Geometry check sheet. Reference: drawing and pictorial views, mm from the part's lowest x, y, z. A direction names the side the tool comes from. Give positions to 0.01 mm unless a question says otherwise; leave off trailing zeros. Order: outer loops, then holes, each group sorted by start corner. A loop starts at its lowest first (then second) coordinate and runs counter-clockwise, first axis right, second up. Notation, with made-up numbers: (68.5, 74.5) - (88.5, 74.5) arc R23 cw to (88.5, 82.5) - close; hole circle Ø3 at (7, 47). An arc over 180 degrees is marked (long way). Answer in a Markdown table with one row per item.
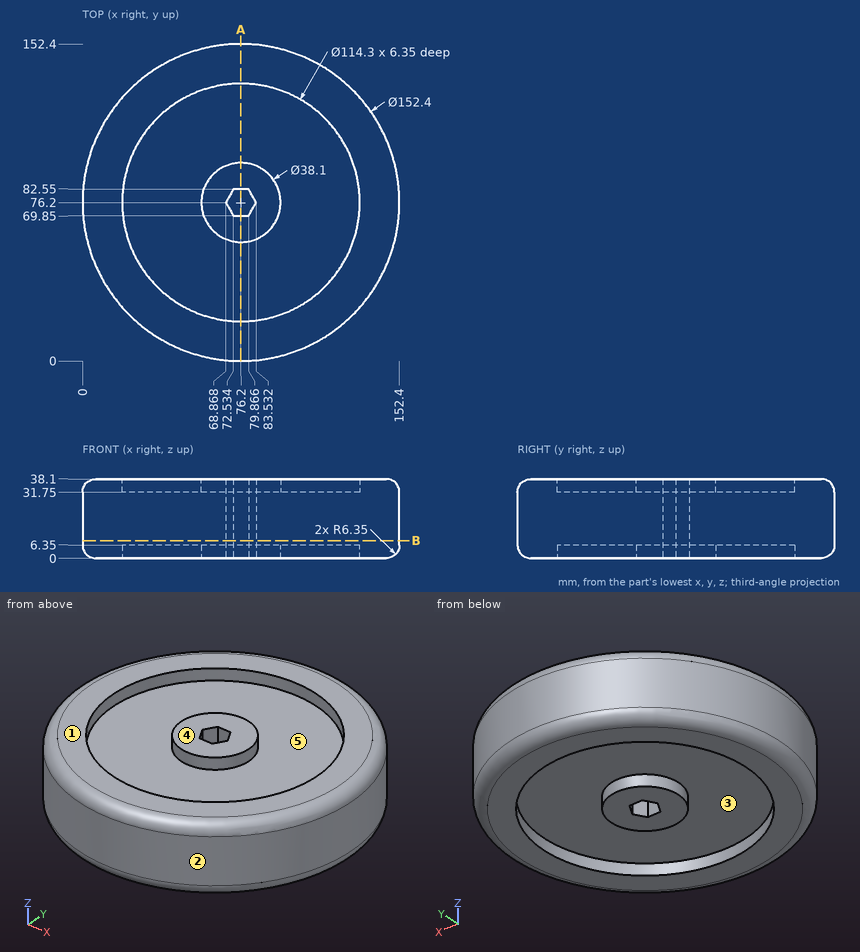
(1) Access from +Z, -Z, +X, -X, +Y, -Y to the whole of each face (thin tool, end or side, straight path). Record for the marked faces 4 and 5.
Geometry says:
| item | result |
|---|---|
| face 4 | +Z, +X, -X, +Y, -Y |
| face 5 | +Z |
(2) Cross-section at A-A, the plane x = 76.2. Record the cut outline in (y, z), then the cut area to 3 significant figures.
Geometry says:
| item | result |
|---|---|
| outline | (0, 6.35) arc R6.35 ccw to (6.35, 0) - (19.05, 0) - (19.05, 6.35) - (57.15, 6.35) - (57.15, 0) - (69.85, 0) - (69.85, 38.1) - (57.15, 38.1) - (57.15, 31.75) - (19.05, 31.75) - (19.05, 38.1) - (6.35, 38.1) arc R6.35 ccw to (0, 31.75) - close; (82.55, 0) - (95.25, 0) - (95.25, 6.35) - (133.35, 6.35) - (133.35, 0) - (146.05, 0) arc R6.35 ccw to (152.4, 6.35) - (152.4, 31.75) arc R6.35 ccw to (146.05, 38.1) - (133.35, 38.1) - (133.35, 31.75) - (95.25, 31.75) - (95.25, 38.1) - (82.55, 38.1) - close |
| area | 4,320 mm² |
(3) Mould release check, pull along X, two halves, no side actions. Record for the marked faces 1, 2 and 3: pulls with the +X half, pulls with the -X half, needs draft (parallel to the pull), parting line crosses it, or undercut.
Geometry says:
| item | result |
|---|---|
| face 1 | needs draft |
| face 2 | parting line crosses it |
| face 3 | undercut |
(4) Cross-section at B-B, the plane z = 8.5. Record the cut outline in (x, y), then the cut area to 3 significant figures.
Geometry says:
| item | result |
|---|---|
| outline | circle Ø152.4 at (76.2, 76.2); hole (68.87, 76.2) - (72.53, 69.85) - (79.87, 69.85) - (83.53, 76.2) - (79.87, 82.55) - (72.53, 82.55) - close |
| area | 18,100 mm² |
(5) Gauge pin test, flat ends, axial feed: P1, Ø8, axis at x = 44, z = 13.5, coming from the +Y side; P2, Ø3, axis at x = 102, y = 119.5, coming from the -Z side; P3, Ø8, axis at x = 92, z = 9.5, coming from the +Y side. Record the tip position at first contact, or that the pin passes through.
Geometry says:
| item | result |
|---|---|
| P1 | y = 146.99 |
| P2 | z = 6.35 |
| P3 | y = 151.48 |
(6) Thickness scan on L1, parallel to Y at x = 76.2, z = 36.25; L2, parallel to X at y = 78, z = 4.5 (1 decimal); L3, parallel to Y at x = 76, z = 36. Record the ranges inside material, lowest first.
Geometry says:
| item | result |
|---|---|
| L1 | 1.87 to 19.05, 57.15 to 69.85, 82.55 to 95.25, 133.35 to 150.53 |
| L2 | 0.3 to 19.1, 57.2 to 69.9, 82.5 to 95.2, 133.3 to 152.1 |
| L3 | 1.63 to 19.05, 57.15 to 69.85, 82.55 to 95.25, 133.35 to 150.77 |
